```python
from build123d import *
from build123d.topology import SkipClean

# Parameters (mm, degrees)
ESBO_O1_R                = 42.5
RESSALTO_EXTRUS_O1_DEPTH = 5
ESBO_O2_R                = 8
RESSALTO_EXTRUS_O2_DEPTH = 8
FILETE3_R                = 15
ESBO_O3_R                = 2.075
CORTE_EXTRUS_O1_DEPTH    = 61.634148794
PADR_OCIRCULAR1_COUNT    = 16
CORTE_EXTRUS_O2_DEPTH    = 61.634148794


with BuildPart() as part:
    # Esboço1 → Ressalto-extrusão1 (new body)
    with BuildSketch(Plane.XY):
        Circle(ESBO_O1_R)
    extrude(amount=RESSALTO_EXTRUS_O1_DEPTH)

    # Esboço2 → Ressalto-extrusão2 (add)
    with BuildSketch(Plane.XY.offset(5)):
        Circle(ESBO_O2_R)
        with BuildLine():
            Line((-2.24624687, 2.1), (2.24624687, 2.1))
            ThreePointArc((2.24624687, 2.1), (0, -3.075), (-2.24624687, 2.1))
        make_face(mode=Mode.SUBTRACT)
    extrude(amount=RESSALTO_EXTRUS_O2_DEPTH)

    # Filete3
    # the kernel refuses this fillet: 15 mm, written as the material it adds along each edge
    with BuildSketch(Plane(origin=(0, 0, 5), x_dir=(1, 0, 0), z_dir=(0, -1, 0))) as filete3_piece_1:
        with BuildLine():
            CenterArc((21.266499161, 15), FILETE3_R, 207.818139285, 62.181860715)
            Line((8, 8), (7.734670017, 7.86))
            ThreePointArc((7.734670017, 7.86), (7.7, 4), (7.7, 0))
            Line((7.7, 0), (8, -0.3))
            Line((8, -0.3), (21.266499161, -0.3))
            Line((21.266499161, -0.3), (21.266499161, 0))
        make_face()
    revolve(axis=Axis((0, 0, 5), (0, 0, 1)))

    # Esboço3 → Corte-extrusão1 (cut, through all)
    with BuildSketch(Plane.XY.offset(5)):
        with Locations((0, 35)):
            Circle(ESBO_O3_R)
    corte_extrus_o1 = extrude(amount=-CORTE_EXTRUS_O1_DEPTH, mode=Mode.SUBTRACT)

    # PadrãoCircular1: Corte-extrusão1 ×16 about axis
    padr_ocircular1_axis = Axis((0, 0, 0), (0, 0, 1))
    for i in range(1, PADR_OCIRCULAR1_COUNT):
        add(corte_extrus_o1.rotate(padr_ocircular1_axis, i * 360 / PADR_OCIRCULAR1_COUNT), mode=Mode.SUBTRACT)

    # Esboço4 → Corte-extrusão2 (cut, through all)
    with SkipClean():  # the faces are left unmerged after this step: merging them gives an invalid solid
        with BuildSketch(Plane.XY.offset(5)):
            with BuildLine():
                Line((2.24624687, 2.1), (-2.24624687, 2.1))
                ThreePointArc((-2.24624687, 2.1), (0, -3.075), (2.24624687, 2.1))
            make_face()
        extrude(amount=-CORTE_EXTRUS_O2_DEPTH, mode=Mode.SUBTRACT)
    add(part.part.scale(1), mode=Mode.REPLACE)  # the faces are merged on a copy


solid = part.part
```
Here's how the part is built. I have some questions about the finished solid (model axes, mm). A direction names the side the tool comes from. Coordinates: 2 decimals unless noted, no trailing zeros. Order: outer loops, then holes, each group sorted by start corner. A loop starts at its lowest first (then second) coordinate and runs counter-clockwise, first axis right, second up.
1) Imagine slicing it at A-A on x = 0. List the corners of the cut face in (y, z) for me (1 decimal), and give its area (3 significant figures).
2) Will these pins go through, and if not, where does the flat tip stop? pin 1 (5 mm diameter, centred on x = 33.5, z = 6.5, fed in from +Y); pin 2 (3.5 mm diameter, centred on x = -1, z = 2, fed in from -Y); pin 3 (1.3 mm diameter, centred on x = -0.5, z = 11, fed in from -Y).
3) We'd pull the mould along Y, two halves only. Please class faces 3 (the face through (3.4, 0.1, 13)), 4 (the face through (-24.66, -26.82, 2.54)), 5 (the face through (34.133, 14.431, 2.535)): +Y half, -Y half, draft (parallel to the pull), parting line (faces both ways), or undercut.
4) Which directions (+Z, -Z, +X, -X, +Y, -Y) give clear straight access to the entire face, cutting with the end or side of a thin tool? Please do faces 1 (the face through (-14.431, 34.133, 2.535)), 2 (the face through (-19, 10, 5)).
5) Imagine slicing it at C-C on z = 1.75. State how many separate pieces and enclosed holes the cut face has, and give its area (3 significant figures).
6) Imagine slicing it at D-D on z = 6.5. List the corners of the cut face in (x, y) for me (3 decimals), and give its area (3 significant figures).
7) I need wall thicknesses on line 1 (X direction, y = -24.5, z = 2); line 2 (X direction, y = 26.5, z = 2.5); line 3 (Y direction, x = -36.5, z = 0.75). Which ranges of each line are inside material? Lowest first, please.
8) Imagine slicing it at B-B on y = 0. List the corners of the cut face in (x, z) for me (1 decimal).
Response values:
1. outline: (-42.5, 0) - (-37.1, 0) - (-37.1, 5) - (-42.5, 5) - close; (-32.9, 0) - (-3.1, 0) - (-3.1, 13) - (-8, 13) arc R15 cw to (-21.3, 5) - (-32.9, 5) - close; (2.1, 0) - (32.9, 0) - (32.9, 5) - (21.3, 5) arc R15 cw to (8, 13) - (2.1, 13) - close; (37.1, 0) - (42.5, 0) - (42.5, 5) - (37.1, 5) - close
1. area: 505 mm2
2. pin 1: stops at y = 28.53
2. pin 2: stops at y = -42.5
2. pin 3: stops at y = -9.77
3. face 3: draft
3. face 4: undercut
3. face 5: undercut
4. face 1: +Z, -Z
4. face 2: +Z
5. separate pieces: 1
5. enclosed holes: 17
5. area: 5,430 mm2
6. outline: circle Ø29.456 at (0, 0); hole (-2.246, 2.1) arc R3.075 ccw (long way) to (2.246, 2.1) - close
6. area: 655 mm2
7. line 1: x = -34.73 to -26.81, -22.69 to 22.69, 26.81 to 34.73
7. line 2: x = -33.23 to -25.86, -23.64 to 23.64, 25.86 to 33.23
7. line 3: y = -21.77 to -1.43, 1.43 to 21.77
8. outline: (-42.5, 0) - (-37.1, 0) - (-37.1, 5) - (-42.5, 5) - close; (-32.9, 0) - (-3.1, 0) - (-3.1, 13) - (-8, 13) arc R15 cw to (-21.3, 5) - (-32.9, 5) - close; (3.1, 0) - (32.9, 0) - (32.9, 5) - (21.3, 5) arc R15 cw to (8, 13) - (3.1, 13) - close; (37.1, 0) - (42.5, 0) - (42.5, 5) - (37.1, 5) - close
